Autodesk Inventor part; units mm, degrees
ref_plane "Work Plane2" through (0, 0, 5) normal (0, 0, 1) x (1, 0, 0)
ref_plane "Work Plane8" through (0, 0, 0) normal (0.9238795, 0.3826834, 0) x (0, 0, 1)
ref_plane "Work Plane9" through (0, 0, 0) normal (1, 0, 0) x (0, 1, 0)
sketch "Sketch1" plane through (0, 0, 0) normal (0, 0, 1) x (1, 0, 0)
  circle A0 centre (0, 0) radius 5
  dimension "d0" = 10
extrude "Extrusion1" add sketch "Sketch1" along normal blind 10
ref_plane "Work Plane2" through (0, 0, 5) normal (0, 0, 1) x (1, 0, 0)
sketch "Sketch2" plane through (0, 0, 0) normal (0, 0, -1) x (-1, 0, 0)
  circle A0 centre (0, 0) radius 5
  circle A1 centre (0, 0) radius 4
  dimension "d3" = 8
surface extrude "Pitch Diameter" sketch "Sketch2" against normal through all shown no curves A1
ref_plane "Work Plane8" through (0, 0, 0) normal (0.9238795, 0.3826834, 0) x (0, 0, 1)
ref_plane "Work Plane9" through (0, 0, 0) normal (1, 0, 0) x (0, 1, 0)
spur gear teeth "Spur Gear" teeth 8 pitch diameter 8 tip diameter 10 root diameter 5.5 face width 10 start plane through (0, 0, 0) normal (0, 0, -1) x (-1, 0, 0)
sketch "Sketch3" plane through (0, 0, 0) normal (0, 0, -1) x (-1, 0, 0)
  point P0 (0, 0)
  point P1 (0, 0)
hole "Hole1" at (0, 0, 0) direction (0, 0, 1) diameter 4 end through all
equation "\"d0\" = da_da"
equation "\"d1\" = da_b"
equation "\"d3\" = da_d"
equation "\"d16\" = da_aw"
equation "\"d43\" = da_aw"
equation "\"d46\" = da_aw"
properties part number "Spur Gear1" material "Steel"
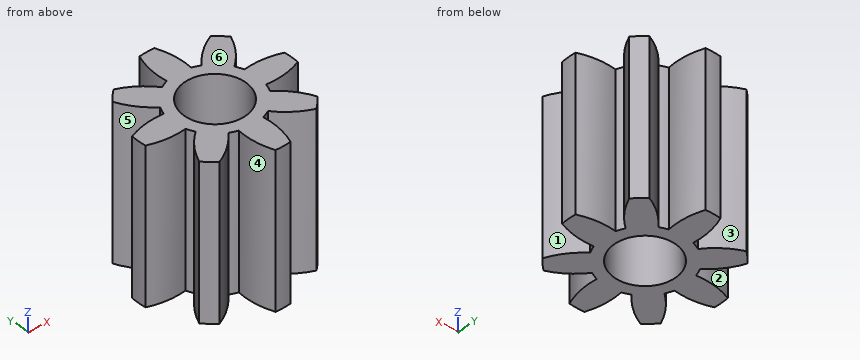
Geometry check sheet. Reference: the model listing, model coordinates, mm. Face numbers are marked on the shaded views. A direction names the side the tool comes from. Give positions to 0.01 mm unless a question says otherwise; leave off trailing zeros. Order: outer loops, then holes, each group sorted by start corner. A loop starts at its lowest first (then second) coordinate and runs counter-clockwise, first axis right, second up. Notation, with made-up numbers: (41.5, 16) - (94.5, 16) arc R21 ccw to (94.5, 41) - close; hole circle Ø6 at (41.25, 33). An arc over 180 degrees is marked (long way). Answer in a Markdown table with one row per item. Add a question column.
Q1. Gauge pin test, flat ends, axial feed: pin 1 (1.5 mm diameter, centred on x = -1, z = 7, fed in from +Y); pin 2 (3 mm diameter, centred on y = -3.5, z = 8.5, fed in from -X); pin 3 (6 mm diameter, centred on y = 4, z = 9, fed in from +X). Record the tip position at first contact, or that the pin passes through.
Q2. Mould release check, pull along X, two halves, no side actions. Record for the marked faces 4, 5 and 6: pulls with the +X half, pulls with the -X half, needs draft (parallel to the pull), parting line crosses it, or undercut.
Q3. Material ranges on probe 1 along Y at (x, z) = (0, 3); probe 2 along X at (y, z) = (3.5, 8), recorded low to high. Write a range as from..to.
Q4. Cross-section at D-D, the plane x = 3.5. Enter the section's corners in (y, z), then the cut area to 3 significant figures.
Q5. Tool access check on the marked faces 1, 2 and 3. Record the directions out of +Z, -Z, +X, -X, +Y, -Y that give a thin tool (end or side, any length) a straight path to the whole face; none if there is none.
Q6. Cross-section at A-A, the plane x = 0. Enter the section's corners in (y, z).
Check values:
| question | item | result |
|---|---|---|
| 1 | pin 1 | stops at y = 4.99 |
| 1 | pin 2 | stops at x = -3.87 |
| 1 | pin 3 | stops at x = 3.87 |
| 2 | face 4 | undercut |
| 2 | face 5 | pulls with the -X half |
| 2 | face 6 | needs draft |
| 3 | probe 1 | y = -5..-2, 2..5 |
| 3 | probe 2 | x = -3.57..-2.48, -0.83..0.83, 2.48..3.57 |
| 4 | outline | (-3.57, 0) - (-2.48, 0) - (-2.48, 10) - (-3.57, 10) - close; (-0.83, 0) - (0.83, 0) - (0.83, 10) - (-0.83, 10) - close; (2.48, 0) - (3.57, 0) - (3.57, 10) - (2.48, 10) - close |
| 4 | area | 38.4 mm^2 |
| 5 | face 1 | +Z, -Z, +X |
| 5 | face 2 | +Z, -Z |
| 5 | face 3 | +Z, -Z, +Y |
| 6 | outline | (-5, 0) - (-2, 0) - (-2, 10) - (-5, 10) - close; (2, 0) - (5, 0) - (5, 10) - (2, 10) - close |
